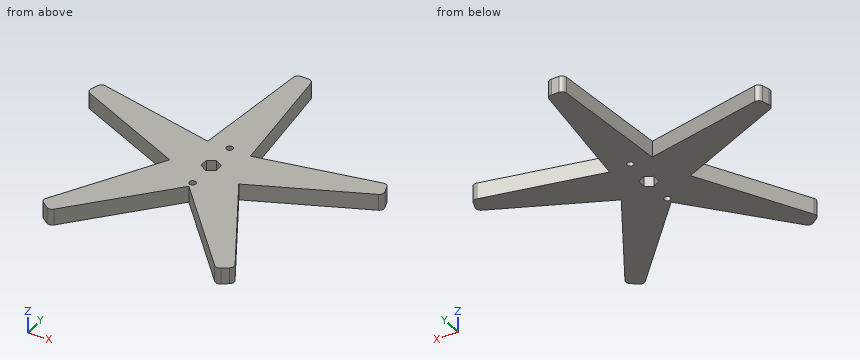
```python
from build123d import *

# Parameters (mm, degrees)
SKETCH1_R           = 2.5
BOSS_EXTRUDE1_DEPTH = 12.7


with BuildPart() as part:
    # Sketch1 → Boss-Extrude1 (new body)
    with BuildSketch(Plane.XY):
        with BuildLine():
            Line((-2.922024956, 118.140407077), (2.922024956, 118.140407077))
            ThreePointArc((2.922024956, 118.140407077), (5.470359591, 117.162736611), (6.710856163, 114.731478252))
            Line((6.710856163, 114.731478252), (16.457987064, 22.652475842))
            Line((16.457987064, 22.652475842), (107.042351415, 41.836380053))
            ThreePointArc((107.042351415, 41.836380053), (109.737950042, 41.407897856), (111.455248619, 39.286404385))
            Line((111.455248619, 39.286404385), (113.261159358, 33.728382634))
            ThreePointArc((113.261159358, 33.728382634), (113.1188182, 31.002655585), (111.189888617, 29.071573086))
            Line((111.189888617, 29.071573086), (26.629582456, -8.652475842))
            Line((26.629582456, -8.652475842), (72.866667573, -88.875173413))
            ThreePointArc((72.866667573, -88.875173413), (73.292142573, -91.571248333), (71.805156827, -93.860073872))
            Line((71.805156827, -93.860073872), (67.077221132, -97.295120224))
            ThreePointArc((67.077221132, -97.295120224), (64.440914824, -98.002041718), (62.008274208, -96.764257979))
            Line((62.008274208, -96.764257979), (0, -28))
            Line((0, -28), (-62.008274208, -96.764257979))
            ThreePointArc((-62.008274208, -96.764257979), (-64.440914824, -98.002041718), (-67.077221132, -97.295120224))
            Line((-67.077221132, -97.295120224), (-71.805156827, -93.860073872))
            ThreePointArc((-71.805156827, -93.860073872), (-73.292142573, -91.571248333), (-72.866667573, -88.875173413))
            Line((-72.866667573, -88.875173413), (-26.629582456, -8.652475842))
            Line((-26.629582456, -8.652475842), (-111.189888617, 29.071573086))
            ThreePointArc((-111.189888617, 29.071573086), (-113.1188182, 31.002655585), (-113.261159358, 33.728382634))
            Line((-113.261159358, 33.728382634), (-111.455248619, 39.286404385))
            ThreePointArc((-111.455248619, 39.286404385), (-109.737950042, 41.407897856), (-107.042351415, 41.836380053))
            Line((-107.042351415, 41.836380053), (-16.457987064, 22.652475842))
            Line((-16.457987064, 22.652475842), (-6.710856163, 114.731478252))
            ThreePointArc((-6.710856163, 114.731478252), (-5.470359591, 117.162736611), (-2.922024956, 118.140407077))
        make_face()
        with Locations((0, 23.341182104)):
            Circle(SKETCH1_R, mode=Mode.SUBTRACT)
        with Locations((0, -23.341182104)):
            Circle(SKETCH1_R, mode=Mode.SUBTRACT)
        Polygon((0, -6.65), (5.759068935, -3.325), (5.759068935, 3.325), (0, 6.65), (-5.759068935, 3.325), (-5.759068935, -3.325), align=None, mode=Mode.SUBTRACT)
    extrude(amount=BOSS_EXTRUDE1_DEPTH)


solid = part.part
```
Work out the finished part from the listing and answer in its coordinate system (mm). Give positions to 0.01 mm unless a question says otherwise; leave off trailing zeros. Write each loop counter-clockwise with the first axis right and the second up, starting at its lowest first coordinate (ties: lowest second). Pieces come first, ordered by that corner, then holes. Notation, with made-up numbers: (27.25, -18) -> (73.25, -18) arc R17 ccw to (73.25, 13) -> close; hole circle Ø6 at (48.25, 74). An arc over 180 degrees is marked (long way). Write item = value, one per line.
Q1. Consider line 1 along Y through (x, z) = (0, 10); line 2 along X through (y, z) = (-88.5, 2.5); line 3 along X through (y, z) = (6, 6.5). Determine where each line is inside the solid, lowest interval first.
Computed values:
line_1 = -28 to -25.84, -20.84 to -6.65, 6.65 to 20.84, 25.84 to 118.14
line_2 = -72.65 to -54.56, 54.56 to 72.65
line_3 = -59.47 to -1.13, 1.13 to 59.47
Q2. Section B-B on z = 4.75 is taken. State how many separate pieces and enclosed holes the cut face has, and give its area (3 significant figures).
Computed values:
separate_pieces = 1
enclosed_holes = 3
area = 12,600 mm^2
Q3. Section A-A on y = -77.5 is taken. Determine the outline of the cut face in (x, z).
Computed values:
outline = (-66.31, 0) -> (-44.64, 0) -> (-44.64, 12.7) -> (-66.31, 12.7) -> close; (44.64, 0) -> (66.31, 0) -> (66.31, 12.7) -> (44.64, 12.7) -> close
Q4. Flat-ended cylindrical pins translate along their axes: pin 1 Ø6 at (x, z) = (-47, 9.5) entering from -Y; pin 2 Ø7.5 at (y, z) = (0, 6.5) entering from -X; pin 3 Ø1 at (y, z) = (3, 5.5) entering from +X; pin 4 Ø4.5 at (x, y) = (0, -23.34) entering from -Z. Find the tip coordinate at first contact, or state that the pin passes through.
Computed values:
pin_1 = -83.45
pin_2 = -54.43
pin_3 = 53.87
pin_4 = through
Q5. Section C-C on x = 56 is taken. Determine the outline of the cut face in (y, z).
Computed values:
outline = (-90.1, 0) -> (-59.61, 0) -> (-59.61, 12.7) -> (-90.1, 12.7) -> close; (4.45, 0) -> (31.03, 0) -> (31.03, 12.7) -> (4.45, 12.7) -> close
Q6. Section D-D on x = 11.5 is taken. Determine the outline of the cut face in (y, z), and give its area (3 significant figures).
Computed values:
outline = (-40.75, 0) -> (69.49, 0) -> (69.49, 12.7) -> (-40.75, 12.7) -> close
area = 1,400 mm^2
